Design review of the part built by this model. Coordinates are the model's own, in mm. A direction names the side the tool comes from. Coordinates: 2 decimals unless noted, no trailing zeros. Loops run counter-clockwise (first coordinate to the right, second up) from the corner with the lowest first, then second, coordinate; pieces in that order, holes last. Notation, with made-up numbers: M 34,64 L 67,64 A11 cw 67,83 Z; hole C -1,64.5 d4. An arc over 180 degrees is marked long. One line per item, written item: value.
```python
from build123d import *

# Parameters (mm, degrees)
F1_DEPTH     = 609.6
F3_DEPTH     = 25.4
F5_DEPTH     = 25.4
F7_DEPTH     = 25.4
F9_DEPTH     = 25.4
F10_T1_DEPTH = 521.3263794739
F10_T3_DEPTH = 630.6724176283
F11_SIZE     = 3.175
F12_T1_DEPTH = 279.7873057355
F12_T3_DEPTH = 270.6235437243
F13_SIZE     = 3.175
F14_SIZE     = 3.175


# Not quite as in the source:
# - a fillet or chamfer that OpenCascade refuses, or shapes differently, is made with other operations: its cross-section is extruded or revolved along the edge and cut away or added


with BuildPart() as f1:
    # F0 (on Right) → F1 (new body)
    with BuildSketch(Plane.YZ):
        Polygon((252.7066397959, 237.49), (-243.0247255434, 104.8818597717), (-244.6656554292, 111.0161771021), (-256.93429009, 107.7343173304), (-255.2933602041, 101.6), (-255.2933602041, 75.3069357006), (252.7066397959, 211.1969357006), align=None)
    extrude(amount=F1_DEPTH)

    # F2 (on face) → F3 (join)
    with BuildSketch(Plane(origin=(0, 252.7066397959, 0), x_dir=(-1, 0, 0), z_dir=(0, 1, 0))):
        Polygon((-609.6, 211.1969357006), (-609.6, -30.1030642994), (-584.2, -30.1030642994), (-584.2, 33.3969357006), (-25.4, 33.3969357006), (-25.4, -30.1030642994), (0, -30.1030642994), (0, 211.1969357006), (-25.4, 211.1969357006), (-25.4, 109.5969357006), (-584.2, 109.5969357006), (-584.2, 211.1969357006), align=None)
    extrude(amount=-F3_DEPTH)

    # F4 (on face) → F5 (join)
    with BuildSketch(Plane.XZ.offset(255.2933602041)):
        Polygon((25.4, 101.6), (0, 101.6), (0, -30.1030642994), (25.4, -30.1030642994), (25.4, 33.3969357006), (584.2, 33.3969357006), (584.2, -30.1030642994), (609.6, -30.1030642994), (609.6, 101.6), (584.2, 101.6), (584.2, 84.1969357006), (25.4, 84.1969357006), align=None)
    extrude(amount=-F5_DEPTH)

    # F6 (on face) → F7 (join)
    with BuildSketch(Plane(origin=(0, 0, 0), x_dir=(0, -1, 0), z_dir=(-1, 0, 0))):
        Polygon((229.8933602041, 82.1014357006), (-227.3066397959, 204.4024357006), (-227.3066397959, 178.1093714013), (229.8933602041, 55.8083714013), align=None)
    extrude(amount=-F7_DEPTH)

    # F8 (on face) → F9 (join)
    with BuildSketch(Plane.YZ.offset(609.6)):
        Polygon((227.3066397959, 204.4024357006), (-229.8933602041, 82.1014357006), (-229.8933602041, 55.8083714013), (227.3066397959, 178.1093714013), align=None)
    extrude(amount=-F9_DEPTH)

    # F10: chamfer of 3.175 on 3 edges, made by hand

    # F10_s2 → F10_t1 (cut)
    with BuildSketch(Plane(origin=(0, 303.005458711, 81.0539602052), x_dir=(1, 0, 0), z_dir=(0, -0.9660342253, -0.2584141553))):
        Polygon((0, 160.9454953054), (3.175, 164.1204953054), (0, 164.1204953054), align=None)
        Polygon((609.6, 160.9454953054), (606.425, 164.1204953054), (609.6, 164.1204953054), align=None)
    extrude(amount=F10_T1_DEPTH, mode=Mode.SUBTRACT)

    # F10_s4 → F10_t3 (cut)
    with BuildSketch(Plane.YZ.offset(-10.5362088142)):
        Polygon((252.7066397959, 233.3540544626), (248.711174853, 236.4212131278), (252.7066397959, 237.49), align=None)
    extrude(amount=F10_T3_DEPTH, mode=Mode.SUBTRACT)

    # F11
    f11_edges = [f1.edges().sort_by_distance(p)[0] for p in [
        (609.6, -1.29336, 116.958871),
        (584.2, -1.29336, 116.958871),
        (25.4, -1.29336, 116.958871),
        (0, -1.29336, 116.958871),
        (609.6, -255.29336, 35.748468),
        (609.6, 252.70664, 101.625495),
        (0, -255.29336, 35.748468),
    ]]
    chamfer(f11_edges, length=F11_SIZE)

    # F12: chamfer of 3.175 on 2 edges, made by hand

    # F12_s2 → F12_t1 (cut)
    with BuildSketch(Plane.XY.offset(-38.2681577861)):
        Polygon((3.175, 252.7066397959), (0, 249.5316397959), (0, 252.7066397959), align=None)
    extrude(amount=F12_T1_DEPTH, mode=Mode.SUBTRACT)

    # F12_s4 → F12_t3 (cut)
    with BuildSketch(Plane.XY.offset(-33.6862767805)):
        Polygon((605.1098719395, 252.7066397959), (607.3549359697, 251.7767038262), (606.425, 252.7066397959), align=None)
    extrude(amount=F12_T3_DEPTH, mode=Mode.SUBTRACT)

    # F13
    f13_edges = [f1.edges().sort_by_distance(p)[0] for p in [
        (304.8, 252.70664, 211.196936),
    ]]
    chamfer(f13_edges, length=F13_SIZE)

    # F14
    f14_edges = [f1.edges().sort_by_distance(p)[0] for p in [
        (304.8, -255.29336, 33.396936),
        (304.8, -229.89336, 33.396936),
    ]]
    chamfer(f14_edges, length=F14_SIZE)


solid = f1.part
```
(1) We need section A-A on x = 373. State the section outline as (y, z) points, then the cut area to 3 significant figures.
Reply:
outline: M -256.93,107.73 L -255.29,101.6 L -255.29,36.57 L -252.12,33.4 L -233.07,33.4 L -229.89,36.57 L -229.89,82.1 L 249.64,210.38 L 252.71,214.37 L 252.71,233.35 L 248.71,236.42 L -243.02,104.88 L -244.67,111.02 Z; M 227.31,33.4 L 252.71,33.4 L 252.71,109.6 L 227.31,109.6 Z
area: 16,500 mm2
(2) To check wall thickness, follow line 1 along Y through (x, z) = (400, 49.5); line 2 along Z through (x, y) = (470.5, -202.5); line 3 along Z through (x, y) = (380, 102.5). State the ranges of each line that lie inside material, in increasing order. Write a range as [from, to].
Reply:
line 1: y = [-255.29, -229.89], [227.31, 252.71]
line 2: z = [89.43, 115.72]
line 3: z = [171.02, 197.31]
(3) We need section C-C on z = 68. State the section outline as (x, y) points (3 decimals).
Reply:
outline: M 0,-252.118 L 3.175,-255.293 L 606.425,-255.293 L 609.6,-252.118 L 609.6,-196.604 L 606.425,-184.317 L 587.375,-184.317 L 584.2,-196.604 L 584.2,-229.893 L 25.4,-229.893 L 25.4,-196.604 L 22.225,-184.317 L 3.175,-184.317 L 0,-196.604 Z; M 0,227.307 L 609.6,227.307 L 609.6,249.532 L 607.355,251.777 L 605.11,252.707 L 3.175,252.707 L 0,249.532 Z
(4) Insertion check: pin 1 (5 mm diameter, centred on x = 478.5, y = 11.5, fed in from -Z); pin 2 (1 mm diameter, centred on x = 421.5, z = 61.5, fed in from -Y); pin 3 (21 mm diameter, centred on x = 348, y = -244, fed in from -Z). Each pin has a flat end and moves straight along its axis. Give the tip position at first contact, or say it passes through.
Reply:
pin 1: stops at z = 146.01
pin 2: stops at y = -255.29
pin 3: stops at z = 33.4
(5) We need section D-D on y = -216. State the section outline as (x, z) points (3 decimals), then the cut area to 3 significant figures.
Reply:
outline: M 0,62.811 L 3.175,59.525 L 22.225,59.525 L 25.4,62.811 L 25.4,85.818 L 584.2,85.818 L 584.2,62.811 L 587.375,59.525 L 606.425,59.525 L 609.6,62.811 L 609.6,108.824 L 606.425,112.111 L 3.175,112.111 L 0,108.824 Z
area: 17,300 mm2
(6) Tool access review of faces 5 (the flat face through (585.765, -4.505, 117.766)), 6 (the flat face through (309, 240, 33.397)), 7 (the flat face through (597, -4.5, 116.1)), 8 (the flat face through (25.4, 48, 137)): name each direction out of +Z, -Z, +X, -X, +Y, -Y from which nothing blocks a thin tool from reaching the whole face with its end or side.
Reply:
face 5: -Z
face 6: -Z, +Y, -Y
face 7: -Z, +X, -X
face 8: none
(7) We need section B-B on z = 164. State the section outline as (x, y) points (1 decimal), then the cut area to 3 significant figures.
Reply:
outline: M 0,-9.7 L 3.2,-22 L 606.4,-22 L 609.6,-9.7 L 609.6,162.3 L 606.4,174.6 L 587.4,174.6 L 584.2,162.3 L 584.2,76.3 L 25.4,76.3 L 25.4,162.3 L 22.2,174.6 L 3.2,174.6 L 0,162.3 Z; M 0,227.3 L 25.4,227.3 L 25.4,252.7 L 3.2,252.7 L 0,249.5 Z; M 584.2,227.3 L 609.6,227.3 L 609.6,249.5 L 607.4,251.8 L 605.1,252.7 L 584.2,252.7 Z
area: 66,100 mm2
(8) Mouldability with a two-part tool opening along Y and no side actions: class faces 1 (the flat face through (303.38, -256.5, 106.11)), 2 (the flat face through (301, -229.893, 64)), 3 (the flat face through (609.6, -5, 132)), 4 (the flat face through (23.83, 1.91, 119.48)) as released by +Y, released by -Y, zero draft, split by the parting line, or undercut.
Reply:
face 1: released by -Y
face 2: undercut
face 3: zero draft
face 4: undercut
